Design review of the part built by this model. Coordinates are the model's own, in mm. Face numbers are marked on the shaded views. Give positions to 0.01 mm unless a question says otherwise; leave off trailing zeros. Order: outer loops, then holes, each group sorted by start corner. A loop starts at its lowest first (then second) coordinate and runs counter-clockwise, first axis right, second up.
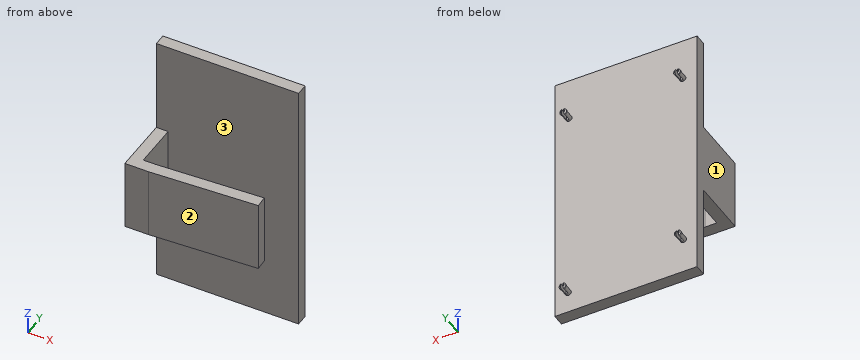
```python
from build123d import *

# Parameters (mm, degrees)
BOSS_EXTRUDE1_DEPTH = 15
SKETCH2_W           = 60
SKETCH2_H           = 110
BOSS_EXTRUDE2_DEPTH = 5
SKETCH3_R           = 1.25
BOSS_EXTRUDE3_DEPTH = 4
SKETCH4_R           = 1.405
BOSS_EXTRUDE4_DEPTH = 1
CHAMFER1_SIZE       = 0.5
SKETCH5_W           = 1
SKETCH5_H           = 3.260897444
CUT_EXTRUDE1_DEPTH  = 4
MIRROR1_START       = 28
MIRROR1_DEPTH       = 6
MIRROR1_2_DEPTH     = 2
MIRROR1_START_2     = 33
MIRROR1_3_DEPTH     = 1
SKETCH7_R           = 1.25
BOSS_EXTRUDE5_DEPTH = 4
SKETCH8_R           = 1.405
BOSS_EXTRUDE6_DEPTH = 1
CHAMFER2_SIZE       = 0.5
SKETCH9_W           = 1
SKETCH9_H           = 4.099421272
SKETCH9_H_2         = 4.814063164
CUT_EXTRUDE2_DEPTH  = 4


with BuildPart() as part:
    # Sketch1 → Boss-Extrude1 (new, symmetric)
    with BuildSketch(Plane.XY):
        Polygon((0, 0), (10, 0), (55, 2.358350068), (54.738678842, 7.344654806), (10, 5), (5, 5), (5, 24), (60, 24), (60, 29), (0, 29), align=None)
    extrude(amount=BOSS_EXTRUDE1_DEPTH, both=True)

    # Sketch2 → Boss-Extrude2 (add)
    with BuildSketch(Plane(origin=(0, 29, 0), x_dir=(1, 0, 0), z_dir=(0, 1, 0))):
        with Locations((30, 0)):
            Rectangle(SKETCH2_W, SKETCH2_H)
    extrude(amount=-BOSS_EXTRUDE2_DEPTH)

    # Sketch3 → Boss-Extrude3 (add)
    with BuildSketch(Plane(origin=(0, 29, 0), x_dir=(1, 0, 0), z_dir=(0, 1, 0))):
        with Locations(Location((54, -37, 0), (0, 0, 90))):
            Circle(SKETCH3_R)
    extrude(amount=BOSS_EXTRUDE3_DEPTH)

    # Sketch4 → Boss-Extrude4 (add)
    with BuildSketch(Plane(origin=(0, 33, 0), x_dir=(1, 0, 0), z_dir=(0, 1, 0))):
        with Locations(Location((54, -37, 0), (0, 0, 270))):
            Circle(SKETCH4_R)
    extrude(amount=BOSS_EXTRUDE4_DEPTH)

    # Chamfer1
    chamfer1_edges = [part.edges().sort_by_distance(p)[0] for p in [
        (54, 34, 35.595),
    ]]
    chamfer(chamfer1_edges, length=CHAMFER1_SIZE)

    # Sketch5 → Cut-Extrude1 (cut)
    with BuildSketch(Plane(origin=(0, 34, 0), x_dir=(1, 0, 0), z_dir=(0, 1, 0))):
        with Locations((54, -37)):
            Rectangle(SKETCH5_W, SKETCH5_H)
    extrude(amount=-CUT_EXTRUDE1_DEPTH, mode=Mode.SUBTRACT)

    # Mirror1: read off the stored shape, not the designer's step
    # Mirror1 outline → Mirror1 (add)
    with BuildSketch(Plane(origin=(0, 0, 0), x_dir=(1, 0, 0), z_dir=(0, 1, 0)).offset(MIRROR1_START)):
        with BuildLine():
            ThreePointArc((6.5, -38.145643924), (7.25, -37), (6.5, -35.854356076))
            Line((6.5, -35.854356076), (6.5, -38.145643924))
        make_face()
        with BuildLine():
            Line((5.5, -38.145643924), (5.5, -35.854356076))
            ThreePointArc((5.5, -35.854356076), (4.75, -37), (5.5, -38.145643924))
        make_face()
    extrude(amount=MIRROR1_DEPTH)

    # Mirror1 2 outline → Mirror1 2 (add)
    with BuildSketch(Plane(origin=(0, 0, 0), x_dir=(1, 0, 0), z_dir=(0, 1, 0)).offset(MIRROR1_START)):
        with BuildLine():
            Line((6.5, -38.145643924), (6.5, -35.854356076))
            ThreePointArc((6.5, -35.854356076), (6, -35.75), (5.5, -35.854356076))
            Line((5.5, -35.854356076), (5.5, -38.145643924))
            ThreePointArc((5.5, -38.145643924), (6, -38.25), (6.5, -38.145643924))
        make_face()
    extrude(amount=MIRROR1_2_DEPTH)

    # Mirror1 3 outline → Mirror1 3 (add)
    with BuildSketch(Plane(origin=(0, 0, 0), x_dir=(1, 0, 0), z_dir=(0, 1, 0)).offset(MIRROR1_START_2)):
        with BuildLine():
            ThreePointArc((6.5, -35.854356076), (7.25, -37), (6.5, -38.145643924))
            Line((6.5, -38.145643924), (6.5, -38.313021325))
            ThreePointArc((6.5, -38.313021325), (7.405, -37), (6.5, -35.686978675))
            Line((6.5, -35.686978675), (6.5, -35.854356076))
        make_face()
        with BuildLine():
            ThreePointArc((5.5, -38.145643924), (4.75, -37), (5.5, -35.854356076))
            Line((5.5, -35.854356076), (5.5, -35.686978675))
            ThreePointArc((5.5, -35.686978675), (4.595, -37), (5.5, -38.313021325))
            Line((5.5, -38.313021325), (5.5, -38.145643924))
        make_face()
    extrude(amount=MIRROR1_3_DEPTH)

    # Mirror1 4 outline → Mirror1 4 (revolve, cut)
    with BuildSketch(Plane(origin=(6, 0, 37), x_dir=(1, 0, 0), z_dir=(0, 0, 1))):
        Polygon((1.405000007, 34.00000007), (0.90499993, 34.00000007), (1.405000007, 33.499999993), align=None)
    revolve(axis=Axis((6, 0, 37), (0, 1, 0)), mode=Mode.SUBTRACT)

    # Sketch7 → Boss-Extrude5 (add)
    with BuildSketch(Plane(origin=(0, 29, 0), x_dir=(1, 0, 0), z_dir=(0, 1, 0))):
        with Locations(Location((54.3, 46, 0), (0, 0, 90))):
            Circle(SKETCH7_R)
        with Locations(Location((5.7, 40, 0), (0, 0, 90))):
            Circle(SKETCH7_R)
    extrude(amount=BOSS_EXTRUDE5_DEPTH)

    # Sketch8 → Boss-Extrude6 (add)
    with BuildSketch(Plane(origin=(0, 33, 0), x_dir=(1, 0, 0), z_dir=(0, 1, 0))):
        with Locations(Location((5.7, 40, 0), (0, 0, 270))):
            Circle(SKETCH8_R)
        with Locations(Location((54.3, 46, 0), (0, 0, 270))):
            Circle(SKETCH8_R)
    extrude(amount=BOSS_EXTRUDE6_DEPTH)

    # Chamfer2
    chamfer2_edges = [part.edges().sort_by_distance(p)[0] for p in [
        (5.7, 34, -41.405),
        (54.3, 34, -47.405),
    ]]
    chamfer(chamfer2_edges, length=CHAMFER2_SIZE)

    # Sketch9 → Cut-Extrude2 (cut)
    with BuildSketch(Plane(origin=(0, 34, 0), x_dir=(1, 0, 0), z_dir=(0, 1, 0))):
        with Locations((5.7, 40)):
            Rectangle(SKETCH9_W, SKETCH9_H)
        with Locations((54.3, 46)):
            Rectangle(SKETCH9_W, SKETCH9_H_2)
    extrude(amount=-CUT_EXTRUDE2_DEPTH, mode=Mode.SUBTRACT)


solid = part.part
```
1. For line 1 along Y through (x, z) = (35, 6); line 2 along Z through (x, y) = (24, 5.5); line 3 along X through (y, z) = (21, -11.5), list the stretches that pass through material, from the lowest coordinate up.
Recorded:
line 1: y = 1.31 to 6.31, 24 to 29
line 2: z = -15 to 15
line 3: x = 0 to 5
2. Draft analysis for pull direction Y (two halves, no side actions). For the marked faces 1, 2 and 3, state which applies: pulls with the +Y half, pulls with the -Y half, needs draft (parallel to the pull), parting line crosses it, or undercut.
Recorded:
face 1: needs draft
face 2: pulls with the -Y half
face 3: undercut
3. For pin 1 (0.5 mm diameter, centred on x = 7, z = 37, fed in from -Y); pin 2 (6 mm diameter, centred on y = 19.5, z = 10.5, fed in from +X); pin 3 (8 mm diameter, centred on y = 27.5, z = 4, fed in from -X); pin 4 (1.5 mm diameter, centred on y = 4.5, z = -7, fed in from +X), all flat-tipped, find the tip position at first contact; note any pin that passes through.
Recorded:
pin 1: stops at y = 24
pin 2: stops at x = 5
pin 3: stops at x = 0
pin 4: stops at x = 54.93
4. Take a section at B-B (z = 9.5). State the section outline as (x, y) points, then the cut area to 3 significant figures.
Recorded:
outline: (0, 0) - (10, 0) - (55, 2.36) - (54.74, 7.34) - (10, 5) - (5, 5) - (5, 24) - (60, 24) - (60, 29) - (0, 29) - close
area: 669 mm2
5. Take a section at C-C (z = -17). State the section outline as (x, y) points.
Recorded:
outline: (0, 24) - (60, 24) - (60, 29) - (0, 29) - close
6. Take a section at A-A (x = 21.5). State the section outline as (y, z) points, then the cut area to 3 significant figures.
Recorded:
outline: (0.6, -15) - (5.6, -15) - (5.6, 15) - (0.6, 15) - close; (24, -55) - (29, -55) - (29, 55) - (24, 55) - close
area: 700 mm2
